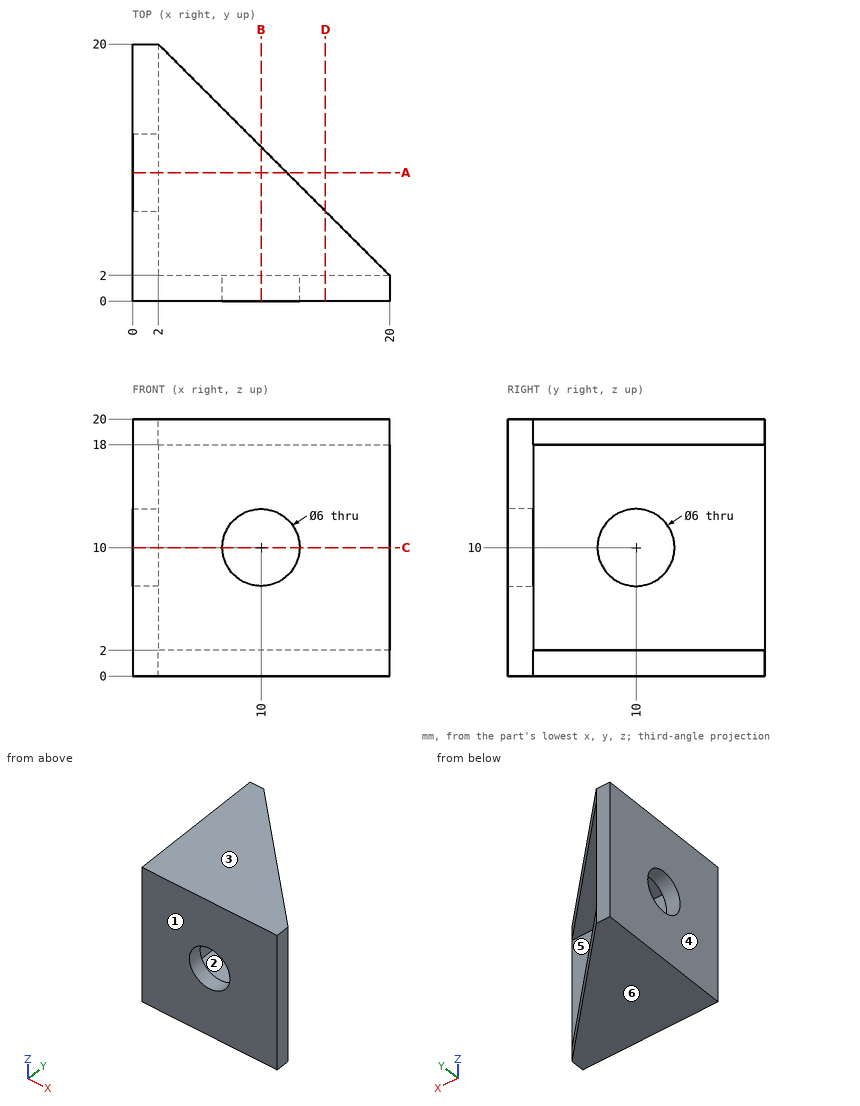
Can you work these out from the drawing? Everything is in mm from the part's minimum corner. A direction names the side the tool comes from. Round coordinates to 2 decimals unless told otherwise and drop trailing zeros. Order: outer loops, then holes, each group sorted by start corner. A loop starts at its lowest first (then second) coordinate and runs counter-clockwise, first axis right, second up.
(1) If I drill on L1, parallel to Y at x = 0.8, z = 10; L2, parallel to Z at x = 4.5, y = 5.75, over which ranges is the centre line in solid material (lowest first)?
Results are:
L1: y = 0 to 7, 13 to 20
L2: z = 0 to 2, 18 to 20
(2) If we section it at A-A (y = 10): Please give me the cut outline in (x, z), plus the area to 3 significant figures.
Results are:
outline: (0, 0) - (12, 0) - (12, 2) - (2, 2) - (2, 7) - (0, 7) - close; (0, 13) - (2, 13) - (2, 18) - (12, 18) - (12, 20) - (0, 20) - close
area: 68.0 mm2
(3) If we section it at D-D (x = 15): Please give me the cut outline in (y, z), plus the area to 3 significant figures.
Results are:
outline: (0, 0) - (7, 0) - (7, 2) - (2, 2) - (2, 18) - (7, 18) - (7, 20) - (0, 20) - close
area: 60.0 mm2
(4) On a 3-axis mill with a long thin cutter (end or side, diameter ignored), from which of +Z, -Z, +X, -X, +Y, -Y can I reach the whole of each face in a straight line? I mean the marked faces 1 and 2. Say none if no direction works.
Results are:
face 1: +Z, -Z, +X, -X, -Y
face 2: +X, +Y
(5) We'd pull the mould along Z, two halves only. Please class the marked faces 3, 4, 5 and 6: +Z half, -Z half, draft (parallel to the pull), parting line (faces both ways), or undercut.
Results are:
face 3: +Z half
face 4: draft
face 5: undercut
face 6: -Z half
(6) If we section it at C-C (z = 10): Please give me the cut outline in (x, y).
Results are:
outline: (0, 0) - (7, 0) - (7, 2) - (2, 2) - (2, 7) - (0, 7) - close; (0, 13) - (2, 13) - (2, 20) - (0, 20) - close; (13, 0) - (20, 0) - (20, 2) - (13, 2) - close
(7) I'm going to push flat-ended pins straight in: pin 1 (12 mm diameter, centred on y = 5.5, z = 6, fed in from -X); pin 2 (4 mm diameter, centred on y = 15.5, z = 8, fed in from +X). Where does each tip first touch, or does it pass through?
Results are:
pin 1: stops at x = 0
pin 2: stops at x = 2
